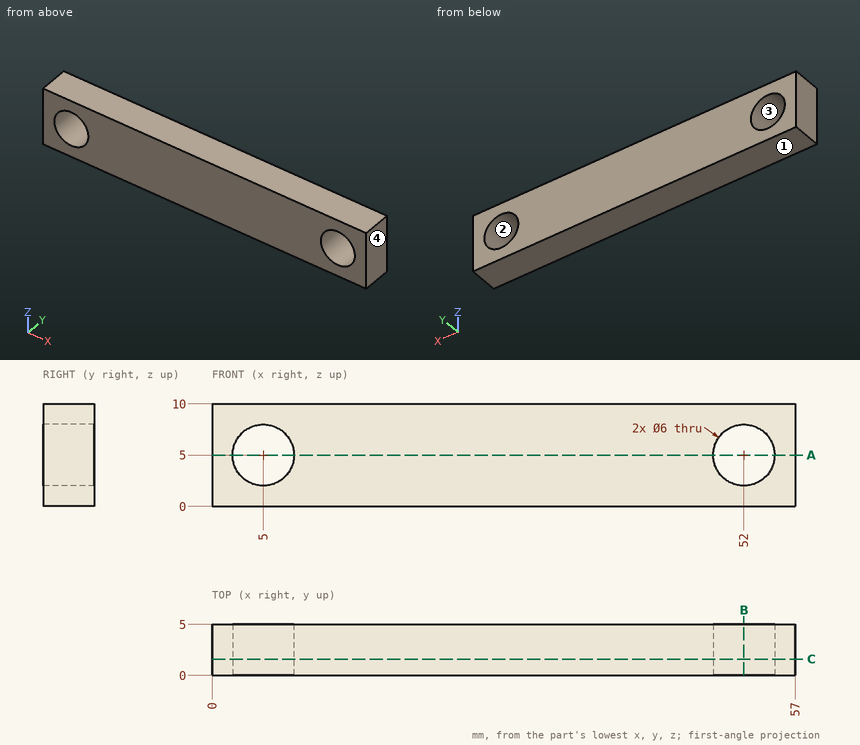
The drawing under review shows one solid part. Ordinate dimensions are in mm from its lowest x, y, z. Give positions to 0.01 mm unless a question says otherwise; leave off trailing zeros. Loops run counter-clockwise (first coordinate to the right, second up) from the corner with the lowest first, then second, coordinate; pieces in that order, holes last. Notation, with made-up numbers: M -32.75,77 L 16.25,77 A36 cw 16.25,115 Z; hole C 70.5,-6.5 d9. An arc over 180 degrees is marked long. Return JSON: item names as keys, results as strings. Group by question number.
Item 1: Insertion check: pin 1 Ø3 at (x, z) = (9, 3.5) entering from -Y; pin 2 Ø3.5 at (x, z) = (52, 5) entering from +Y. Each pin has a flat end and moves straight along its axis. Give the tip position at first contact, or say it passes through.
Item 2: We need section B-B (x = 52). Give the boundary of the cut face in (y, z).
Item 3: We need section C-C (y = 1.6). Give the boundary of the cut face in (x, z).
Item 4: For probe 1 along X at (y, z) = (3.5, 5); probe 2 along X at (y, z) = (1.65, 5.75); probe 3 along Z at (x, y) = (53.5, 4), list the stretches that pass through material, from the lowest coordinate up.
Item 5: Mouldability with a two-part tool opening along Z and no side actions: class the marked faces 1, 2, 3 and 4 as released by +Z, released by -Z, zero draft, split by the parting line, or undercut.
Item 6: We need section A-A (z = 5). Give the boundary of the cut face in (x, y), and give its area (3 significant figures).
Output:
{
 "1": {"pin 1": "stops at y = 0", "pin 2": "passes through"},
 "2": {"outline": "M 0,0 L 5,0 L 5,2 L 0,2 Z; M 0,8 L 5,8 L 5,10 L 0,10 Z"},
 "3": {"outline": "M 0,0 L 57,0 L 57,10 L 0,10 Z; hole C 5,5 d6; hole C 52,5 d6"},
 "4": {"probe 1": "x = 0 to 2, 8 to 49, 55 to 57", "probe 2": "x = 0 to 2.1, 7.9 to 49.1, 54.9 to 57", "probe 3": "z = 0 to 2.4, 7.6 to 10"},
 "5": {"face 1": "released by -Z", "face 2": "undercut", "face 3": "undercut", "face 4": "zero draft"},
 "6": {"outline": "M 0,0 L 2,0 L 2,5 L 0,5 Z; M 8,0 L 49,0 L 49,5 L 8,5 Z; M 55,0 L 57,0 L 57,5 L 55,5 Z", "area": "225 mm^2"}
}
